Part model, mm, in its own coordinate system. Give positions to 0.01 mm unless a question says otherwise; leave off trailing zeros. Write each loop counter-clockwise with the first axis right and the second up, starting at its lowest first coordinate (ties: lowest second). Pieces come first, ordered by that corner, then holes. Notation, with made-up numbers: M 63.5,-31.5 L 76.5,-31.5 A6 ccw 76.5,-25.5 Z; hole C 33,47 d3. An arc over 180 degrees is marked long. Use CSV: the item, a comma, the result in double quotes. Start each with the question number.
1. Drop flat-ended pins along their axis: pin 1 Ø3 at (x, y) = (18.575, 298.5) entering from +Z; pin 2 Ø0.5 at (x, z) = (2.5, 4) entering from +Y. Give the stop position or say it passes through.
2. Band-saw the part on B-B, the plane z = 3.9. Count the separate pieces of the cut face and the enclosed holes in it, then the cut area to 3 significant figures.
3. Band-saw the part on A-A, the plane y = 173.5. List the corners of the cut face in (x, z), then the cut area to 3 significant figures.
4. Drill centre lines: line 1 along X through (y, z) = (193.5, 2.8) (3 decimals); line 2 along X through (y, z) = (71, 3.25); line 3 along X through (y, z) = (276, 1.95). Where is each one in solid material? Low to high. Write a range as from..to.
from build123d import *

# Parameters (mm, degrees)
ESQUISSE1_W             = 45
ESQUISSE1_H             = 343.5
ESQUISSE1_R             = 2
ESQUISSE1_W_2           = 5
ESQUISSE1_H_2           = 6
BOSS_EXTRU_1_DEPTH      = 6
ESQUISSE2_W             = 6
ESQUISSE2_H             = 6
BOSS_EXTRU_2_DEPTH      = 6
ENL_V_MAT_EXTRU_1_DEPTH = 351.274892049
ESQUISSE4_R             = 2
ENL_V_MAT_EXTRU_2_DEPTH = 6


with BuildPart() as part:
    # Esquisse1 → Boss.-Extru.1 (new body)
    with BuildSketch(Plane.XY):
        with Locations((0, 171.75)):
            Rectangle(ESQUISSE1_W, ESQUISSE1_H)
        with Locations((0, 70.5)):
            Circle(ESQUISSE1_R, mode=Mode.SUBTRACT)
        with Locations((-18, 70.5)):
            Rectangle(ESQUISSE1_W_2, ESQUISSE1_H_2, mode=Mode.SUBTRACT)
        with Locations((-8, 70.5)):
            Rectangle(ESQUISSE1_W_2, ESQUISSE1_H_2, mode=Mode.SUBTRACT)
        with Locations((8, 70.5)):
            Rectangle(ESQUISSE1_W_2, ESQUISSE1_H_2, mode=Mode.SUBTRACT)
        with Locations((18, 70.5)):
            Rectangle(ESQUISSE1_W_2, ESQUISSE1_H_2, mode=Mode.SUBTRACT)
    extrude(amount=BOSS_EXTRU_1_DEPTH)

    # Esquisse2 → Boss.-Extru.2 (add)
    with BuildSketch(Plane(origin=(0, 343.5, 0), x_dir=(1, 0, 0), z_dir=(0, 1, 0))):
        with Locations((-19.5, -3)):
            Rectangle(ESQUISSE2_W, ESQUISSE2_H)
        with Locations((19.5, -3)):
            Rectangle(ESQUISSE2_W, ESQUISSE2_H)
        with Locations((7.5, -3)):
            Rectangle(ESQUISSE2_W, ESQUISSE2_H)
        with Locations((-7.5, -3)):
            Rectangle(ESQUISSE2_W, ESQUISSE2_H)
    boss_extru_2 = extrude(amount=BOSS_EXTRU_2_DEPTH)

    # Esquisse3 → Enlèv. mat.-Extru.1 (cut, through all)
    with BuildSketch(Plane.XY.offset(6)):
        Polygon((-2, 343.5), (2, 343.5), (2, 337.5), (3, 337.5), (3, 334.5), (2, 334.5), (2, 329.5), (-2, 329.5), (-2, 334.5), (-3, 334.5), (-3, 337.5), (-2, 337.5), align=None)
    enl_v_mat_extru_1 = extrude(amount=-ENL_V_MAT_EXTRU_1_DEPTH, mode=Mode.SUBTRACT)

    # Symétrie1: Boss.-Extru.2, Enlèv. mat.-Extru.1 across plane
    add(boss_extru_2.mirror(Plane.ZX.offset(171.75)))
    add(enl_v_mat_extru_1.mirror(Plane.ZX.offset(171.75)), mode=Mode.SUBTRACT)

    # Esquisse4 → Enlèv. mat.-Extru.2 (cut)
    with BuildSketch(Plane.XY.offset(6)):
        with Locations((-18.575, 88.5)):
            Circle(ESQUISSE4_R)
        with Locations((18.575, 88.5)):
            Circle(ESQUISSE4_R)
        with Locations((-18.575, 103.5)):
            Circle(ESQUISSE4_R)
        with Locations((18.575, 103.5)):
            Circle(ESQUISSE4_R)
        with Locations((-18.575, 118.5)):
            Circle(ESQUISSE4_R)
        with Locations((18.575, 118.5)):
            Circle(ESQUISSE4_R)
        with Locations((-18.575, 133.5)):
            Circle(ESQUISSE4_R)
        with Locations((18.575, 133.5)):
            Circle(ESQUISSE4_R)
        with Locations((-18.575, 148.5)):
            Circle(ESQUISSE4_R)
        with Locations((18.575, 148.5)):
            Circle(ESQUISSE4_R)
        with Locations((-18.575, 163.5)):
            Circle(ESQUISSE4_R)
        with Locations((18.575, 163.5)):
            Circle(ESQUISSE4_R)
        with Locations((-18.575, 178.5)):
            Circle(ESQUISSE4_R)
        with Locations((18.575, 178.5)):
            Circle(ESQUISSE4_R)
        with Locations((-18.575, 193.5)):
            Circle(ESQUISSE4_R)
        with Locations((18.575, 193.5)):
            Circle(ESQUISSE4_R)
        with Locations((-18.575, 208.5)):
            Circle(ESQUISSE4_R)
        with Locations((18.575, 208.5)):
            Circle(ESQUISSE4_R)
        with Locations((-18.575, 223.5)):
            Circle(ESQUISSE4_R)
        with Locations((18.575, 223.5)):
            Circle(ESQUISSE4_R)
        with Locations((-18.575, 238.5)):
            Circle(ESQUISSE4_R)
        with Locations((18.575, 238.5)):
            Circle(ESQUISSE4_R)
        with Locations((-18.575, 253.5)):
            Circle(ESQUISSE4_R)
        with Locations((18.575, 253.5)):
            Circle(ESQUISSE4_R)
        with Locations((-18.575, 268.5)):
            Circle(ESQUISSE4_R)
        with Locations((18.575, 268.5)):
            Circle(ESQUISSE4_R)
        with Locations((-18.575, 283.5)):
            Circle(ESQUISSE4_R)
        with Locations((18.575, 283.5)):
            Circle(ESQUISSE4_R)
        with Locations((-18.575, 298.5)):
            Circle(ESQUISSE4_R)
        with Locations((18.575, 298.5)):
            Circle(ESQUISSE4_R)
        with Locations((-18.575, 313.5)):
            Circle(ESQUISSE4_R)
        with Locations((18.575, 313.5)):
            Circle(ESQUISSE4_R)
        with BuildLine():
            Line((-5, 83.5), (-5, 309.5))
            ThreePointArc((-5, 309.5), (0, 314.5), (5, 309.5))
            Line((5, 309.5), (5, 83.5))
            ThreePointArc((5, 83.5), (0, 78.5), (-5, 83.5))
        make_face()
    extrude(amount=-ENL_V_MAT_EXTRU_2_DEPTH, mode=Mode.SUBTRACT)


solid = part.part
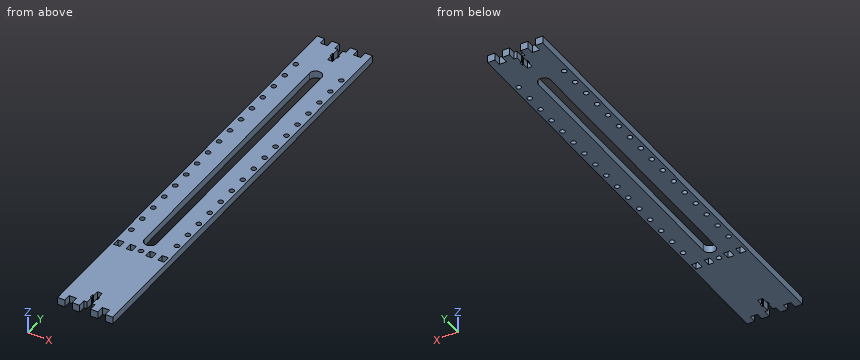
Output:
1,pin 1,"passes through"
1,pin 2,"stops at y = 343.5"
2,separate pieces,"1"
2,enclosed holes,"38"
2,area,"12,700 mm²"
3,outline,"M -22.5,0 L -5,0 L -5,6 L -22.5,6 Z; M 5,0 L 22.5,0 L 22.5,6 L 5,6 Z"
3,area,"210 mm²"
4,line 1,"x = -22.5..-20.575, -16.575..-5, 5..16.575, 20.575..22.5"
4,line 2,"x = -22.5..-20.5, -15.5..-10.5, -5.5..-1.94, 1.94..5.5, 10.5..15.5, 20.5..22.5"
4,line 3,"x = -22.5..-5, 5..22.5"
